Could you check a few things on this model? Use its own coordinates, in mm. Face numbers are marked on the shaded views. A direction names the side the tool comes from. Coordinates: 2 decimals unless noted, no trailing zeros. Order: outer loops, then holes, each group sorted by start corner. A loop starts at its lowest first (then second) coordinate and runs counter-clockwise, first axis right, second up. Notation, with made-up numbers: (-37.75, 19.5) - (8.25, 19.5) arc R32 ccw to (8.25, 58.5) - close; hole circle Ø1 at (29, 58). An arc over 180 degrees is marked (long way). One line per item, written item: value.
Autodesk Inventor part; units mm, degrees
ref_plane "Work Plane1" through (29, 0, 0) normal (0, -1, 0) x (1, 0, 0)
ref_plane "YZ Plane" through (0, 0, 0) normal (1, 0, 0) x (0, 1, 0)
ref_plane "XZ Plane" through (0, 0, 0) normal (0, 1, 0) x (-1, 0, 0)
sketch "Sketch1" plane through (0, 0, 0) normal (0, 0, 1) x (1, 0, 0)
  line L0 (-2.6667, 0) -> (30, 0)
  line L1 (30, 0) -> (30, 6)
  line L2 (30, 6) -> (4.375, 6)
  line L3 (4.375, 6) -> (3.3014, 6)
  line L4 (3.3014, 6) -> (0, 6)
  line L5 (0, 6) -> (0, 9)
  line L6 (0, 9) -> (-12, 9)
  line L7 (-12, 9) -> (-12, 5.7735)
  line L8 (-12, 5.7735) -> (-6, 5.7735)
  line L9 (-6, 5.7735) -> (-2.6667, 0)
  line L10 (-20.4, 0) -> (38.4, 0)
  line L11 (0, -1.8) -> (0, 10.8)
  line L12 (4.375, 6) -> (0, 6) construction
  dimension "d1" = 25.625
  dimension "d2" = 1.0736
  dimension "d3" = 12
  dimension "d4" = 6
  dimension "d5" = 60
  dimension "d6" = 12
  dimension "d7" = 12
  dimension "d8" = 11.547
  dimension "d9" = 18
  dimension "d26" = 30
revolve "Body" add sketch "Sketch1" angle 360 about axis through (-2.6667, 0, 0) along (1, 0, 0)
sketch "Sketch2" plane through (-12, 0, 0) normal (-1, 0, 0) x (0, 0, 1)
  circle A0 centre (0, 0) radius 5.7735
  line L0 (0, -12.6) -> (0, 12.6)
  line L1 (-12.6, 0) -> (12.6, 0)
  line L2 (5.7735, 0) -> (2.8868, -5)
  line L3 (2.8868, -5) -> (-2.8868, -5)
  line L4 (-2.8868, -5) -> (-5.7735, 0)
  line L5 (-5.7735, 0) -> (-2.8868, 5)
  line L6 (-2.8868, 5) -> (2.8868, 5)
  line L7 (2.8868, 5) -> (5.7735, 0)
extrude "Slot" add sketch "Sketch2" against normal up to next contours L7 A0 | A0 L2 | L6 L0 A0 | A0 L0 L3 | L0 L6 A0 | A0 L3 L0 | L4 A0 | A0 L5
fillet "Fillet1" radius 1.2 1 edges at (-12, -9, 0)
thread "Thread"
chamfer "Chamfer1" distance 1.0735 distance2 1.0735 1 edges at (30, -6, 0) measured on face at (30, 0.7092, -1.4219)
ref_plane "Work Plane1" through (29, 0, 0) normal (0, -1, 0) x (1, 0, 0)
fillet "Fillet2" radius 0.1 1 edges at (0, -6, 0)
equation "\"d1\" = GEL"
equation "\"d3\" = KOH"
equation "\"d4\" = INTI"
equation "\"d6\" = GD"
equation "\"d7\" = BDM"
equation "\"d8\" = 1.1547 * SW"
equation "\"d9\" = KOD"
equation "\"d26\" = NLG"
equation "\"d30\" = R"
equation "\"d17\" = RR"
equation "\"d13\" = GEL"
equation "\"d15\" = -0.5 * SPD + 0.5 * GD"
equation "\"d16\" = GUL"
equation "\"GD\" = NND"
equation "\"NLG\" = 30"
equation "\"GEL\" = 25.625"
equation "\"KOD\" = 18"
equation "\"KOH\" = NND"
equation "\"INTI\" = 6"
equation "\"GAL\" = 0.61345 * PTC"
equation "\"GUL\" = 0.61345 * PTC"
equation "\"BDM\" = NND"
equation "\"RR\" = 0.1 * NND"
equation "\"SPD\" = NND - 1.2269 * PTC"
equation "\"R\" = 0.1"
equation "\"PHH\" = 0.25"
equation "\"GD1\" = THREADDIA - 1.2269 * PTC"
equation "\"THREADDIA\" = 12"
equation "\"FAWI\" = 45deg"
equation "\"PTC\" = 1.75"
equation "\"KOH1\" = 10.8"
equation "\"NND\" = 12"
equation "\"TOA\" = 30deg"
equation "\"E0\" = 1.155 * SW"
properties part number "AS 1420 - 1973 - M12 x 30" material "Steel, Mild"
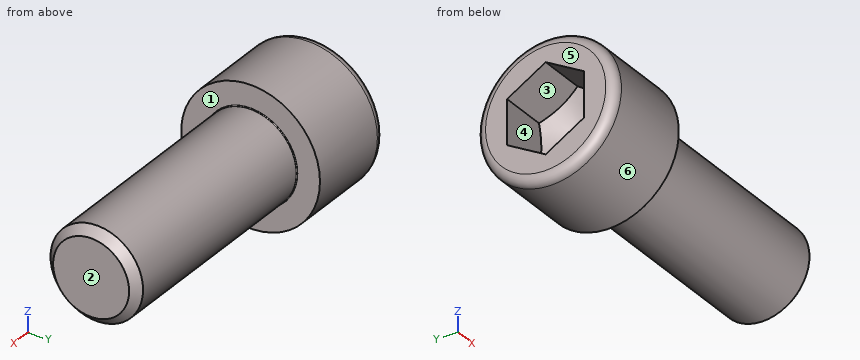
Item 1: I'm going to push flat-ended pins straight in: pin 1 Ø8 at (x, y) = (12, 3) entering from -Z; pin 2 Ø5 at (x, y) = (24.5, 6.5) entering from -Z; pin 3 Ø2 at (x, y) = (19.5, -3) entering from -Z. Where does each tip first touch, or does it pass through?
Conclusion:
pin 1: z = -6
pin 2: z = -4.47
pin 3: z = -5.66
Item 2: For the marked faces 1, 2 and 3, which set-ups out of +Z, -Z, +X, -X, +Y, -Y let a thin tool reach every point of the face, with its end or its side?
Conclusion:
face 1: +X
face 2: +Z, -Z, +X, +Y, -Y
face 3: -X
Item 3: If I drill on probe 1 along X at (y, z) = (7.5, 1.75); probe 2 along Y at (x, z) = (-5, -1); probe 3 along X at (y, z) = (0.5, 0), over which ranges is the centre line in solid material (lowest first)?
Conclusion:
probe 1: -12 to 0
probe 2: -8.94 to -3.92, 3.92 to 8.94
probe 3: -2.96 to 30
Item 4: Thinking about a two-plate mould opening in Z: for the marked faces 4, 5 and 6, which applies, pulls with the +Z half, pulls with the -Z half, needs draft (parallel to the pull), parting line crosses it, or undercut?
Conclusion:
face 4: undercut
face 5: needs draft
face 6: parting line crosses it
Item 5: I want a section at A-A on x = 2.5. Please give me the cut outline in (y, z).
Conclusion:
outline: circle Ø12 at (0, 0)
